Could you check a few things on this drawing? It's one solid part, dimensions in mm from its lowest x, y, z. A direction names the side the tool comes from. Round coordinates to 2 decimals unless told otherwise and drop trailing zeros. Write each loop counter-clockwise with the first axis right and the second up, starting at its lowest first coordinate (ties: lowest second). Pieces come first, ordered by that corner, then holes. Notation, with made-up numbers: M -3,-21.75 L 14,-21.75 A18 cw 14,11.25 Z; hole C -24,69 d9. An arc over 180 degrees is marked long. One line per question, with ' | ' between items. Start each with the question number.
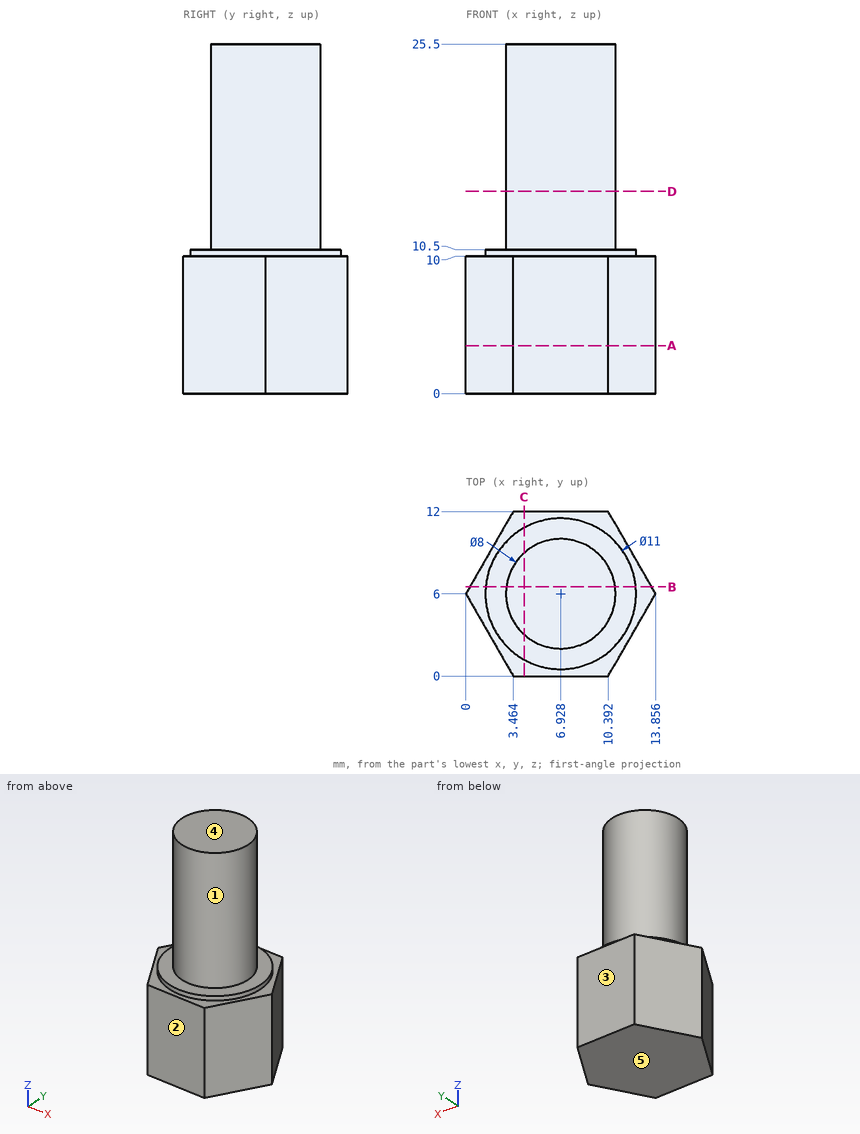
1. Suppose I cut it at A-A (z = 3.5). Write out the boundary of the cut face in (x, y), and give its area (3 significant figures).
2. I need wall thicknesses on line 1 along Z through (x, y) = (11, 5.75); line 2 along Z through (x, y) = (11.5, 2.25); line 3 along X through (y, z) = (3.75, 2.5). Which ranges of each line are inside material? Lowest first, please. Write a range as from..to.
3. Suppose I cut it at B-B (y = 6.5). Write out the boundary of the cut face in (x, z) (1 decimal).
4. Suppose I cut it at D-D (z = 14.75). Write out the boundary of the cut face in (x, y).
5. Suppose I cut it at C-C (x = 4.25). Write out the boundary of the cut face in (y, z).
6. I'm going to push flat-ended pins straight in: P1, Ø1.5, axis at y = 2.5, z = 16, coming from the +X side; P2, Ø2, axis at x = 12, z = 16.5, coming from the +Y side; P3, Ø4, axis at x = 10.5, z = 16.5, coming from the +Y side. Where does each tip first touch, or does it pass through?
7. Which directions (+Z, -Z, +X, -X, +Y, -Y) give clear straight access to the entire face, cutting with the end or side of a thin tool? Please do the marked faces 1 and 2.
8. If we mould it in two halves opening along Z, with no side actions, what happens to the marked faces 3, 4 and 5? For each: released by +Z, released by -Z, zero draft, split by the parting line, or undercut.
Computed:
1) outline: M 0,6 L 3.46,0 L 10.39,0 L 13.86,6 L 10.39,12 L 3.46,12 Z | area: 125 mm²
2) line 1: z = 0..10.5 | line 2: z = 0..10 | line 3: x = 1.3..12.56
3) outline: M 0.3,0 L 13.6,0 L 13.6,10 L 12.4,10 L 12.4,10.5 L 10.9,10.5 L 10.9,25.5 L 3,25.5 L 3,10.5 L 1.5,10.5 L 1.5,10 L 0.3,10 Z
4) outline: C 6.93,6 d8
5) outline: M 0,0 L 12,0 L 12,10 L 10.8,10 L 10.8,10.5 L 8.97,10.5 L 8.97,25.5 L 3.03,25.5 L 3.03,10.5 L 1.2,10.5 L 1.2,10 L 0,10 Z
6) P1: stops at x = 9.83 | P2: passes through | P3: stops at y = 9.68
7) face 1: +Z | face 2: +Z, -Z, +X, -X, -Y
8) face 3: zero draft | face 4: released by +Z | face 5: released by -Z
